Input: part model. Units: mm. Frame: model coordinates. A direction names the side the tool comes from. Round coordinates to 2 decimals unless told otherwise and drop trailing zeros. Loops run counter-clockwise (first coordinate to the right, second up) from the corner with the lowest first, then second, coordinate; pieces in that order, holes last. Notation, with made-up numbers: (7.25, 25) -> (58.25, 25) arc R30 cw to (58.25, 52) -> close; hole circle Ø10 at (8.5, -6). An arc over 180 degrees is marked (long way). Answer in a Markdown table with one row per item. Add a question column.
Q1. Section C-C, the plane x = 3.1. Output: boundary loops of the cut face in (y, z).
Q2. Section A-A, the plane y = 3.5. Output: boundary loops of the cut face in (x, z).
Q3. Pin query (flat end, axial travel): pin 1 (1.5 mm diameter, centred on y = 4.5, z = 44.5, fed in from +X); pin 2 (0.5 mm diameter, centred on x = 4, z = 27.5, fed in from -Y); pin 3 (0.5 mm diameter, centred on x = 0.5, z = 63, fed in from -Y); pin 4 (3 mm diameter, centred on x = 2.5, z = 85, fed in from +Y). Return the tip coordinate at first contact, or that it passes through.
Q4. Ray query, L1, parallel to Z at x = 2.85, y = 0.5; L2, parallel to Y at x = 3, z = 77.5; L3, parallel to X at y = 2.25, z = 85. Return the intervals inside material, ascending. Write a range as from..to.
Q5. Section B-B, the plane z = 45. Output: boundary loops of the cut face in (x, y), and give its area (3 significant figures).
Q6. Mould query, pull axis Y, two halves, no side actions, for faces 1 (the face through (3, -1, 2)), 2 (the face through (4, 4, 20)), 3 (the face through (2.54, 3.57, 14)). Classes: pulls with the +Y half, pulls with the -Y half, needs draft (parallel to the pull), parting line crosses it, or undercut.
Q7. Section D-D, the plane z = 16. Output: boundary loops of the cut face in (x, y), and give its area (3 significant figures).
Q8. Reachability of faces 4 (the face through (1, 7, 44)), 5 (the face through (4, 4, 70)) from +Z, -Z, +X, -X, +Y, -Y: full face, straight path, thin tool, end or side. Return the list, or none.
```python
from build123d import *

# Parameters (mm, degrees)
MAIN_DEPTH               = 90
ESQUISSE2_R              = 1.5
HOLESFORPOWERBOARD_DEPTH = 6
ESQUISSE4_R              = 1.6
HOLESFORMAKERBEAM_DEPTH  = 9
SKETCH1_W                = 50
SKETCH1_H                = 5
POWERBOARDPINHOLES_DEPTH = 3
SKETCH2_R                = 1.25
WINDOWFIXHOLES_DEPTH     = 6


with BuildPart() as part:
    # Esquisse1 → Main (new body)
    with BuildSketch(Plane.XY):
        Polygon((0, 7), (5, 7), (5, 0), (3.95, 0), (3.95, -1), (1.05, -1), (1.05, 0), (0, 0), align=None)
    extrude(amount=MAIN_DEPTH)

    # Esquisse2 → HolesForPowerBoard (cut, through all)
    with BuildSketch(Plane(origin=(5, 0, 0), x_dir=(0, 0, -1), z_dir=(1, 0, 0))):
        with Locations((-12.5, 3.5)):
            Circle(ESQUISSE2_R)
        with Locations((-77.5, 3.5)):
            Circle(ESQUISSE2_R)
    extrude(amount=-HOLESFORPOWERBOARD_DEPTH, mode=Mode.SUBTRACT)

    # Esquisse4 → HolesForMakerBeam (cut, through all)
    with BuildSketch(Plane(origin=(0, -1, 0), x_dir=(-1, 0, 0), z_dir=(0, -1, 0))):
        with Locations((-2.5, -85)):
            Circle(ESQUISSE4_R)
        with Locations((-2.5, -5)):
            Circle(ESQUISSE4_R)
    extrude(amount=-HOLESFORMAKERBEAM_DEPTH, mode=Mode.SUBTRACT)

    # Sketch1 → PowerBoardPinHoles (cut)
    with BuildSketch(Plane(origin=(5, 0, 0), x_dir=(0, 0, -1), z_dir=(1, 0, 0))):
        with Locations((-45, 4.5)):
            Rectangle(SKETCH1_W, SKETCH1_H)
    extrude(amount=-POWERBOARDPINHOLES_DEPTH, mode=Mode.SUBTRACT)

    # Sketch2 → WindowFixHoles (cut, through all)
    with BuildSketch(Plane.ZY):
        with Locations((45, 3.5)):
            Circle(SKETCH2_R)
    extrude(amount=-WINDOWFIXHOLES_DEPTH, mode=Mode.SUBTRACT)


solid = part.part
```
Answer block:
| question | item | result |
|---|---|---|
| 1 | outline | (-1, 0) -> (7, 0) -> (7, 3.52) -> (-1, 3.52) -> close; (-1, 6.48) -> (7, 6.48) -> (7, 20) -> (2, 20) -> (2, 70) -> (7, 70) -> (7, 83.52) -> (-1, 83.52) -> close; (-1, 86.48) -> (7, 86.48) -> (7, 90) -> (-1, 90) -> close; hole circle Ø3 at (3.5, 12.5); hole circle Ø3 at (3.5, 77.5) |
| 2 | outline | (0, 0) -> (5, 0) -> (5, 11) -> (0, 11) -> close; (0, 14) -> (5, 14) -> (5, 20) -> (2, 20) -> (2, 43.75) -> (0, 43.75) -> close; (0, 46.25) -> (2, 46.25) -> (2, 70) -> (5, 70) -> (5, 76) -> (0, 76) -> close; (0, 79) -> (5, 79) -> (5, 90) -> (0, 90) -> close; hole circle Ø3.2 at (2.5, 5); hole circle Ø3.2 at (2.5, 85) |
| 3 | pin 1 | x = 2 |
| 3 | pin 2 | y = -1 |
| 3 | pin 3 | y = 0 |
| 3 | pin 4 | through |
| 4 | L1 | 0..3.44, 6.56..83.44, 86.56..90 |
| 4 | L2 | -1..2, 5..7 |
| 4 | L3 | 0..0.9, 4.1..5 |
| 5 | outline | (0, 0) -> (1.05, 0) -> (1.05, -1) -> (3.95, -1) -> (3.95, 0) -> (5, 0) -> (5, 2) -> (2, 2) -> (2, 2.25) -> (0, 2.25) -> close; (0, 4.75) -> (2, 4.75) -> (2, 7) -> (0, 7) -> close |
| 5 | area | 17.9 mm^2 |
| 6 | face 1 | pulls with the -Y half |
| 6 | face 2 | needs draft |
| 6 | face 3 | undercut |
| 7 | outline | (0, 0) -> (1.05, 0) -> (1.05, -1) -> (3.95, -1) -> (3.95, 0) -> (5, 0) -> (5, 7) -> (0, 7) -> close |
| 7 | area | 37.9 mm^2 |
| 8 | face 4 | +Z, -Z, +X, -X, +Y |
| 8 | face 5 | +X, +Y |
